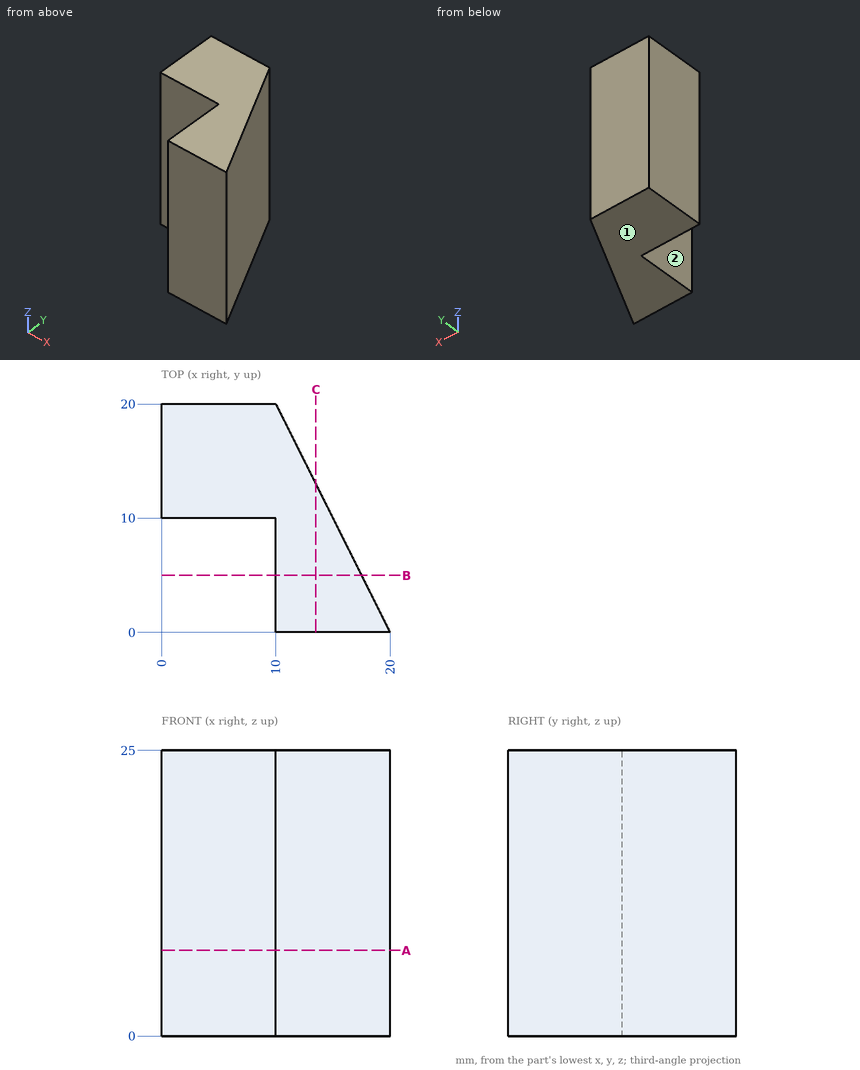
Check sheet for the drawn part. Datum: minimum x, y, z corner. Units: mm. A direction names the side the tool comes from. Round coordinates to 2 decimals unless told otherwise and drop trailing zeros. Write each loop counter-clockwise with the first axis right and the second up, starting at its lowest first coordinate (ties: lowest second). Pieces come first, ordered by that corner, then holes. Notation, with made-up numbers: (11.5, 46) -> (67.5, 46) arc R21 ccw to (67.5, 68) -> close; hole circle Ø6 at (4.5, 57.5). An arc over 180 degrees is marked (long way). Write each question's results on one line, items separated by ' | '.
Q1. Sectioned sample at A-A, the plane z = 7.5. Record the boundary of the cut face in (x, y).
Derived:
outline: (0, 10) -> (10, 10) -> (10, 0) -> (20, 0) -> (10, 20) -> (0, 20) -> close
Q2. Thickness scan on probe 1 along Y at (x, z) = (7.25, 6.5); probe 2 along X at (y, z) = (13.5, 21.25); probe 3 along Y at (x, z) = (14.5, 9.5). Record the ranges inside material, lowest first.
Derived:
probe 1: y = 10 to 20 | probe 2: x = 0 to 13.25 | probe 3: y = 0 to 11
Q3. Access from +Z, -Z, +X, -X, +Y, -Y to the whole of each face (thin tool, end or side, straight path). Record for the marked faces 1 and 2.
Derived:
face 1: -Z, +X, -X, +Y, -Y | face 2: +Z, -Z, -X, -Y
Q4. Sectioned sample at C-C, the plane x = 13.5. Record the boundary of the cut face in (y, z).
Derived:
outline: (0, 0) -> (13, 0) -> (13, 25) -> (0, 25) -> close
Q5. Go/stop test with flat-tipped pins: pin 1 Ø8 at (y, z) = (12.5, 15) entering from -X; pin 2 Ø5 at (y, z) = (15, 13) entering from +X; pin 3 Ø8 at (y, z) = (14, 13.5) entering from +X; pin 4 Ø8 at (x, z) = (3.5, 21) entering from -Y. Record where each tip stops, or that it passes through.
Derived:
pin 1: stops at x = 0 | pin 2: stops at x = 13.75 | pin 3: stops at x = 15 | pin 4: stops at y = 10
Q6. Sectioned sample at B-B, the plane y = 5. Record the boundary of the cut face in (x, z), and give its area (4 significant figures).
Derived:
outline: (10, 0) -> (17.5, 0) -> (17.5, 25) -> (10, 25) -> close | area: 187.5 mm²
